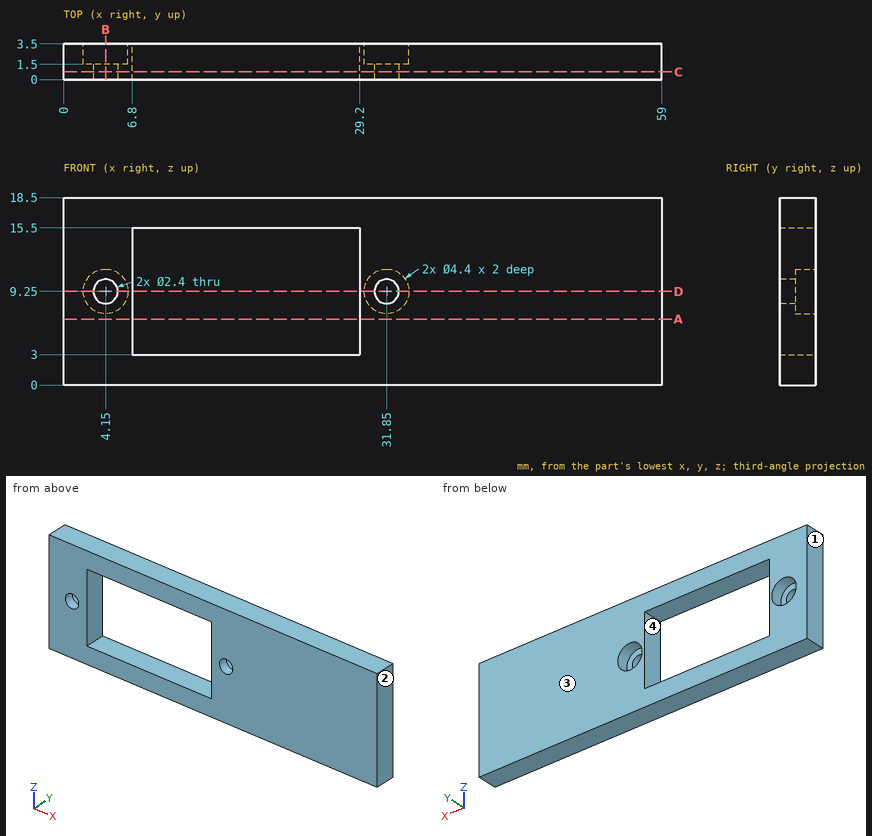
Design review of the part shown in the three views and the two pictorial views. Dimensions are in mm from the part's minimum x, y and z. Coordinates: 2 decimals unless noted, no trailing zeros. Order: outer loops, then holes, each group sorted by start corner. A loop starts at its lowest first (then second) coordinate and runs counter-clockwise, first axis right, second up. Notation, with made-up numbers: (89, -11.75) - (118, -11.75) arc R8 cw to (118, -4.75) - close; hole circle Ø10 at (-1.75, 5). An arc over 180 degrees is marked (long way). Answer as CSV lines item,"result". Start each with the question number.
1) To check wall thickness, follow line 1 along X through (y, z) = (2.65, 9.25); line 2 along X through (y, z) = (1, 9.25); line 3 along Z through (x, y) = (31.85, 0.45). State the ranges of each line that lie inside material, in increasing order. Write a range as [from, to].
2) Draft analysis for pull direction X (two halves, no side actions). For the marked faces 1, 2, 3 and 4, state which applies: +X half, -X half, draft (parallel to the pull), parting line (faces both ways), or undercut.
3) Add section B-B (x = 4.15). State the section outline as (y, z) points, then the cut area to 4 significant figures.
4) Add section D-D (z = 9.25). State the section outline as (x, y) points, then the cut area to 3 significant figures.
5) Insertion check: P1, Ø2, axis at x = 4.15, z = 9.25, coming from the +Y side. The pin has a flat end and moves straight along its axis. Give the tip position at first contact, or say it passes through.
6) Add section C-C (y = 0.75). State the section outline as (x, z) points.
7) Add section A-A (z = 6.5). State the section outline as (x, y) points.
Result:
1,line 1,"[0, 1.95], [6.35, 6.8], [29.2, 29.65], [34.05, 59]"
1,line 2,"[0, 2.95], [5.35, 6.8], [29.2, 30.65], [33.05, 59]"
1,line 3,"[0, 8.05], [10.45, 18.5]"
2,face 1,"-X half"
2,face 2,"+X half"
2,face 3,"draft"
2,face 4,"undercut"
3,outline,"(0, 0) - (3.5, 0) - (3.5, 7.05) - (1.5, 7.05) - (1.5, 8.05) - (0, 8.05) - close; (0, 10.45) - (1.5, 10.45) - (1.5, 11.45) - (3.5, 11.45) - (3.5, 18.5) - (0, 18.5) - close"
3,area,"52.35 mm^2"
4,outline,"(0, 0) - (2.95, 0) - (2.95, 1.5) - (1.95, 1.5) - (1.95, 3.5) - (0, 3.5) - close; (5.35, 0) - (6.8, 0) - (6.8, 3.5) - (6.35, 3.5) - (6.35, 1.5) - (5.35, 1.5) - close; (29.2, 0) - (30.65, 0) - (30.65, 1.5) - (29.65, 1.5) - (29.65, 3.5) - (29.2, 3.5) - close; (33.05, 0) - (59, 0) - (59, 3.5) - (34.05, 3.5) - (34.05, 1.5) - (33.05, 1.5) - close"
4,area,"103 mm^2"
5,P1,"through"
6,outline,"(0, 0) - (59, 0) - (59, 18.5) - (0, 18.5) - close; hole circle Ø2.4 at (4.15, 9.25); hole (6.8, 3) - (29.2, 3) - (29.2, 15.5) - (6.8, 15.5) - close; hole circle Ø2.4 at (31.85, 9.25)"
7,outline,"(0, 0) - (6.8, 0) - (6.8, 3.5) - (0, 3.5) - close; (29.2, 0) - (59, 0) - (59, 3.5) - (29.2, 3.5) - close"
